The listing builds one solid part. Answer for the finished solid, in the listing's coordinates (mm). Face numbers are marked on the shaded views. A direction names the side the tool comes from. Coordinates: 2 decimals unless noted, no trailing zeros. Loops run counter-clockwise (first coordinate to the right, second up) from the corner with the lowest first, then second, coordinate; pieces in that order, holes last. Notation, with made-up numbers: M 4.25,-4 L 60.25,-4 A11 ccw 60.25,2 Z; hole C -24.75,2.25 d9. An arc over 180 degrees is marked long. Answer in a Markdown table with one row per item. Add a question column.
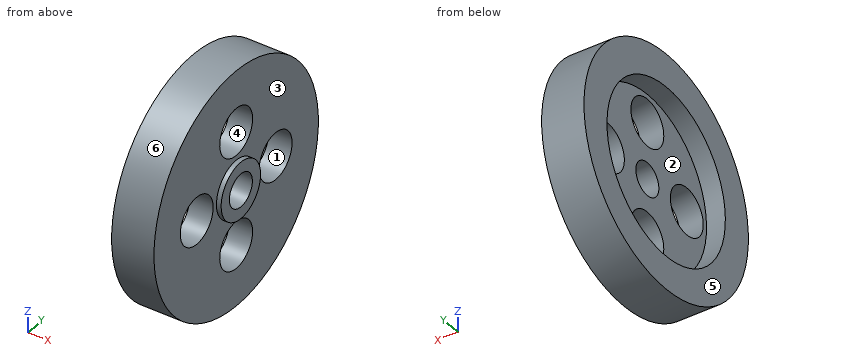
from build123d import *

# Parameters (mm, degrees)
SKETCH1_R           = 25
SKETCH1_R_2         = 3.5
BOSS_EXTRUDE1_DEPTH = 10
CUT_EXTRUDE2_START  = -1
SKETCH2_R           = 25
SKETCH2_R_2         = 6
CUT_EXTRUDE2_DEPTH  = 1
SKETCH3_R           = 5
CUT_EXTRUDE3_DEPTH  = 37.482872694
SKETCH4_R           = 18
CUT_EXTRUDE4_DEPTH  = 4


with BuildPart() as part:
    # Sketch1 → Boss-Extrude1 (new body)
    with BuildSketch(Plane(origin=(0, 0, 0), x_dir=(0, 0, -1), z_dir=(1, 0, 0))):
        Circle(SKETCH1_R)
        Circle(SKETCH1_R_2, mode=Mode.SUBTRACT)
    extrude(amount=BOSS_EXTRUDE1_DEPTH)

    # Sketch2 → Cut-Extrude2 (cut)
    with BuildSketch(Plane(origin=(10, 0, 0), x_dir=(0, 0, -1), z_dir=(1, 0, 0)).offset(CUT_EXTRUDE2_START)):
        Circle(SKETCH2_R)
        Circle(SKETCH2_R_2, mode=Mode.SUBTRACT)
    extrude(amount=CUT_EXTRUDE2_DEPTH, mode=Mode.SUBTRACT)

    # Sketch3 → Cut-Extrude3 (cut, through all)
    with BuildSketch(Plane(origin=(9, 0, 0), x_dir=(0, 0, -1), z_dir=(1, 0, 0))):
        with Locations((0, 12)):
            Circle(SKETCH3_R)
        with Locations((12, 0)):
            Circle(SKETCH3_R)
        with Locations((0, -12)):
            Circle(SKETCH3_R)
        with Locations((-12, 0)):
            Circle(SKETCH3_R)
    extrude(amount=-CUT_EXTRUDE3_DEPTH, mode=Mode.SUBTRACT)

    # Sketch4 → Cut-Extrude4 (cut)
    with BuildSketch(Plane.ZY):
        Circle(SKETCH4_R)
    extrude(amount=-CUT_EXTRUDE4_DEPTH, mode=Mode.SUBTRACT)


solid = part.part
(1) For the marked faces 1, 2 and 3, determine the directions among +Z, -Z, +X, -X, +Y, -Y from which every point of the face is accessible in a straight line to the end or side of a thin tool.
(2) A cutting plane is placed at D-D (z = -12). Give the vertices of the cut face in (x, y), plus the area to 3 significant figures.
(3) Straight lines are drawn through the part: line 1 (Y direction, x = 7.3, z = 0); line 2 (Z direction, x = 4.5, y = -1); line 3 (Y direction, x = 2.1, z = 0). For each, find the intervals that lie inside material, in ascending order.
(4) A cutting plane is placed at B-B (y = 13.5). Give the vertices of the cut face in (x, z).
(5) Each of these flat-tipped pins is pushed along its axis until it touches: pin 1 (3 mm diameter, centred on x = 1.5, y = -8.5, fed in from -Z); pin 2 (5 mm diameter, centred on x = 5.5, z = -5, fed in from -Y); pin 3 (11.5 mm diameter, centred on y = 0, z = -12, fed in from -X). Where does it stop, or does it pass through?
(6) A cutting plane is placed at A-A (z = 0). Give the vertices of the cut face in (x, y), plus the area to 3 significant figures.
(7) The mould has two halves that part along Z. Classify the marked faces 4, 5 and 6: released by +Z, released by -Z, zero draft, split by the parting line, or undercut.
(8) A cutting plane is placed at C-C (x = 7.75). Give the vertices of the cut face in (y, z), plus the area to 3 significant figures.
Solved:
| question | item | result |
|---|---|---|
| 1 | face 1 | +X, -X |
| 1 | face 2 | -X |
| 1 | face 3 | +X |
| 2 | outline | M 0,-21.93 L 9,-21.93 L 9,-5 L 4,-5 L 4,-13.42 L 0,-13.42 Z; M 0,13.42 L 4,13.42 L 4,5 L 9,5 L 9,21.93 L 0,21.93 Z |
| 2 | area | 237 mm² |
| 3 | line 1 | y = -25 to -17, -7 to -3.5, 3.5 to 7, 17 to 25 |
| 3 | line 2 | z = -24.98 to -16.9, -7.1 to -3.35, 3.35 to 7.1, 16.9 to 24.98 |
| 3 | line 3 | y = -25 to -18, 18 to 25 |
| 4 | outline | M 0,-21.04 L 9,-21.04 L 9,-4.77 L 4,-4.77 L 4,-11.91 L 0,-11.91 Z; M 0,11.91 L 4,11.91 L 4,4.77 L 9,4.77 L 9,21.04 L 0,21.04 Z |
| 5 | pin 1 | stops at z = -24 |
| 5 | pin 2 | stops at y = -24.87 |
| 5 | pin 3 | stops at x = 4 |
| 6 | outline | M 0,-25 L 9,-25 L 9,-17 L 4,-17 L 4,-18 L 0,-18 Z; M 0,18 L 4,18 L 4,17 L 9,17 L 9,25 L 0,25 Z; M 4,-7 L 9,-7 L 9,-6 L 10,-6 L 10,-3.5 L 4,-3.5 Z; M 4,3.5 L 10,3.5 L 10,6 L 9,6 L 9,7 L 4,7 Z |
| 6 | area | 176 mm² |
| 7 | face 4 | undercut |
| 7 | face 5 | zero draft |
| 7 | face 6 | split by the parting line |
| 8 | outline | C 0,0 d50; hole C -12,0 d10; hole C 0,-12 d10; hole C 0,12 d10; hole C 0,0 d7; hole C 12,0 d10 |
| 8 | area | 1,610 mm² |
